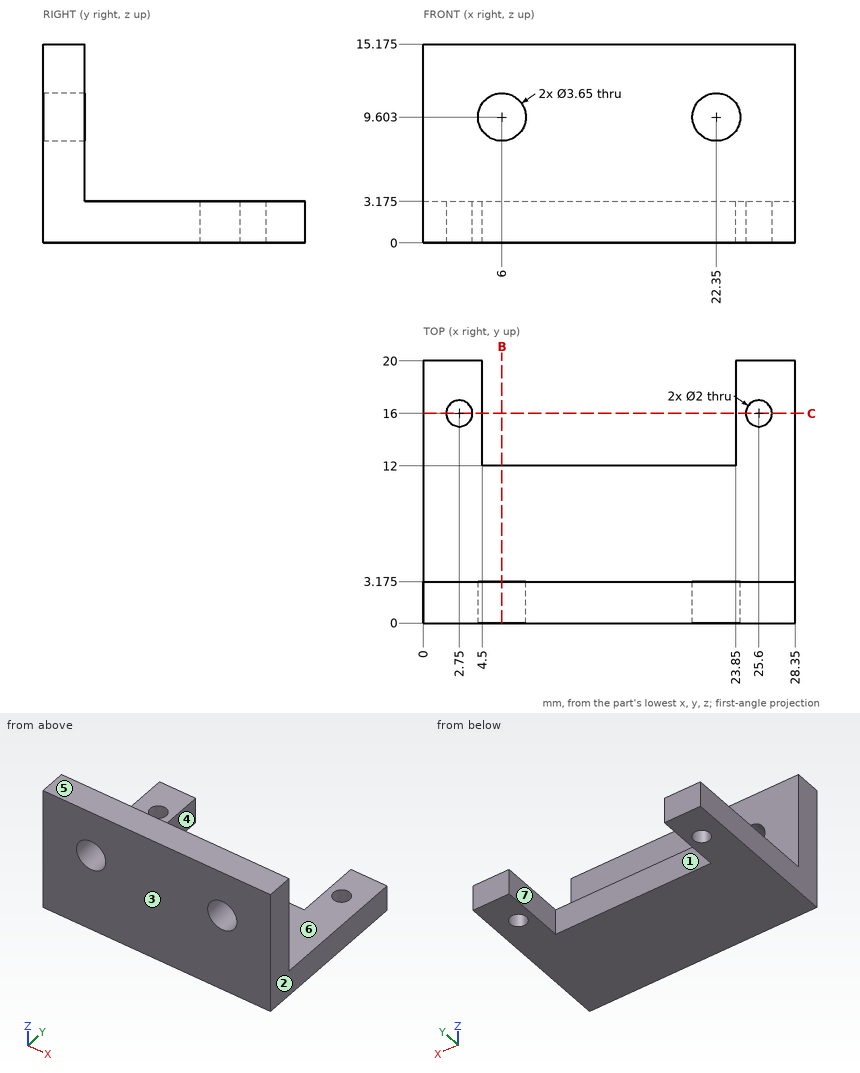
Geometry check sheet. Reference: drawing and pictorial views, mm from the part's lowest x, y, z. A direction names the side the tool comes from. Coordinates: 2 decimals unless noted, no trailing zeros. Order: outer loops, then holes, each group sorted by start corner. A loop starts at its lowest first (then second) coordinate and runs counter-clockwise, first axis right, second up. Notation, with made-up numbers: (36, -10.75) - (79, -10.75) arc R15 ccw to (79, 11.25) - close; hole circle Ø9 at (-24.5, 70.25). An arc over 180 degrees is marked (long way). Answer in a Markdown table with one row per item. Add a question column.
1) Cross-section at C-C, the plane y = 16. State how many separate pieces and enclosed holes the cut face has, then the cut area to 3 significant figures.
2) Cross-section at B-B, the plane x = 6. Record the cut outline in (y, z) (1 decimal), then the cut area to 3 significant figures.
3) Gauge pin test, flat ends, axial feed: P1, Ø8, axis at x = 21, y = 11.5, coming from the +Z side (3 decimals); P2, Ø4.5, axis at x = 6, z = 9.6, coming from the +Y side (3 decimals); P3, Ø2.5, axis at x = 14, z = 1, coming from the +Y side. Record the tip position at first contact, or that the pin passes through.
4) Material ranges on line 1 along X through (y, z) = (2.75, 9.25); line 2 along Y through (x, z) = (25.6, 2.1); line 3 along Y through (x, z) = (19.75, 13.25) (1 decimal), recorded low to high. Write a range as [from, to].
5) Set-up check for the marked faces 5, 6 and 7: record each of +Z, -Z, +X, -X, +Y, -Y from which the full face is reachable in a straight line by a thin tool's end or side.
6) Release check for a two-part mould opening along X. For the marked faces 1, 2, 3 and 4 record: +X half, -X half, draft (parallel to the pull), parting line (faces both ways), or undercut.
Check result:
| question | item | result |
|---|---|---|
| 1 | separate pieces | 4 |
| 1 | enclosed holes | 0 |
| 1 | area | 15.9 mm² |
| 2 | outline | (0, 0) - (12, 0) - (12, 3.2) - (3.2, 3.2) - (3.2, 7.8) - (0, 7.8) - close; (0, 11.4) - (3.2, 11.4) - (3.2, 15.2) - (0, 15.2) - close |
| 2 | area | 64.6 mm² |
| 3 | P1 | stops at z = 3.175 |
| 3 | P2 | stops at y = 3.175 |
| 3 | P3 | stops at y = 12 |
| 4 | line 1 | x = [0, 4.21], [7.79, 20.56], [24.14, 28.35] |
| 4 | line 2 | y = [0, 15], [17, 20] |
| 4 | line 3 | y = [0, 3.2] |
| 5 | face 5 | +Z, +X, -X, +Y, -Y |
| 5 | face 6 | +Z, +X, -X, +Y |
| 5 | face 7 | +Z, -Z, +Y |
| 6 | face 1 | undercut |
| 6 | face 2 | +X half |
| 6 | face 3 | draft |
| 6 | face 4 | undercut |
